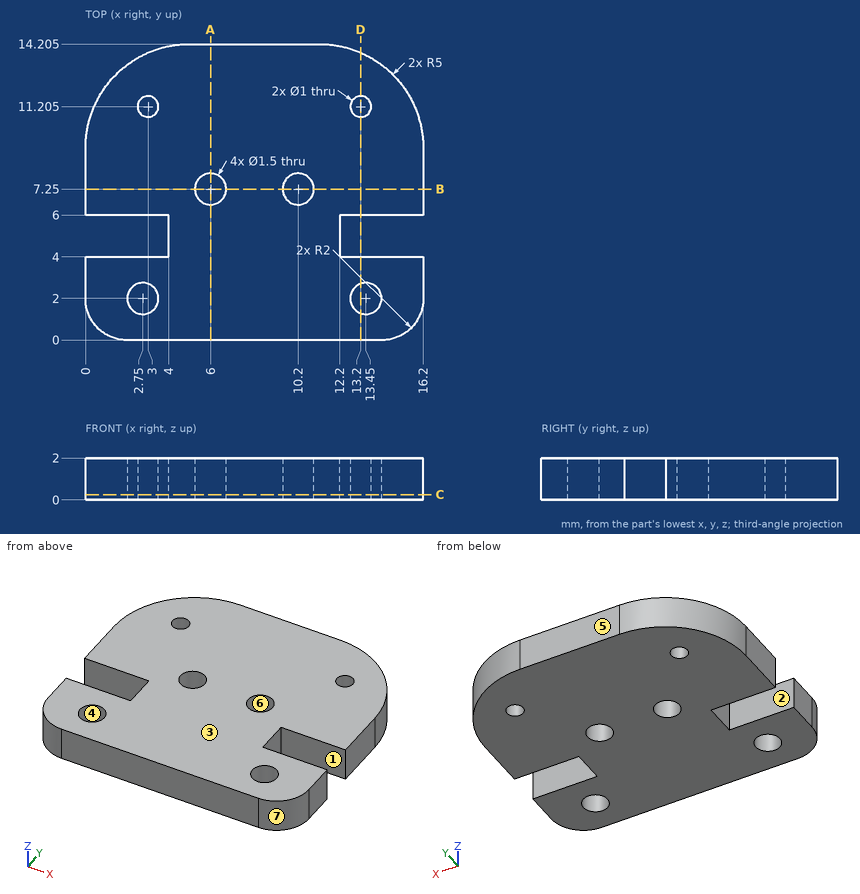
Here's the drawing with two shaded views (mm, measured from the low corner). I have some questions. A direction names the side the tool comes from. Coordinates: 2 decimals unless noted, no trailing zeros. Order: outer loops, then holes, each group sorted by start corner. A loop starts at its lowest first (then second) coordinate and runs counter-clockwise, first axis right, second up. Notation, with made-up numbers: M 5.5,64.25 L 21.5,64.25 A18 ccw 21.5,68.25 Z; hole C 60,61 d3. An arc over 180 degrees is marked long. Write item = value, one per line.
(1) For pin 1 Ø2 at (x, y) = (6, 7.25) entering from +Z; pin 2 Ø1 at (x, z) = (14, 0.5) entering from +Y; pin 3 Ø0.6 at (y, z) = (5, 1.5) entering from +X; pin 4 Ø1 at (x, z) = (3.5, 0.5) entering from +Y, each with a flat end and sliding along its axis, tell me the tip position at first contact or that it passes through.
Results are:
pin_1 = 2
pin_2 = 13.64
pin_3 = 12.2
pin_4 = 14.1
(2) I need wall thicknesses on line 1 along Y through (x, z) = (3, 0.6) (3 decimals); line 2 along Y through (x, z) = (6, 0.7) (3 decimals); line 3 along Y through (x, z) = (1.75, 1.8). Which ranges of each line are inside material? Lowest first, please. Write a range as [from, to].
Results are:
line_1 = [0, 1.293], [2.707, 4], [6, 10.705], [11.705, 13.788]
line_2 = [0, 6.5], [8, 14.205]
line_3 = [0.02, 4], [6, 13]
(3) Suppose I cut it at A-A on x = 6. Please give me the cut outline in (y, z) (3 decimals), plus the area to 3 significant figures.
Results are:
outline = M 0,0 L 6.5,0 L 6.5,2 L 0,2 Z; M 8,0 L 14.205,0 L 14.205,2 L 8,2 Z
area = 25.4 mm2
(4) Suppose I cut it at C-C on z = 0.25. Please give me the cut outline in (x, y) (3 decimals), plus the area to 3 significant figures.
Results are:
outline = M 0,2 A2 ccw 2,0 L 14.2,0 A2 ccw 16.2,2 L 16.2,4 L 12.2,4 L 12.2,6 L 16.2,6 L 16.2,9.205 A5 ccw 11.2,14.205 L 5,14.205 A5 ccw 0,9.205 L 0,6 L 4,6 L 4,4 L 0,4 Z; hole C 2.75,2 d1.5; hole C 3,11.205 d1; hole C 6,7.25 d1.5; hole C 10.2,7.25 d1.5; hole C 13.45,2 d1.5; hole C 13.2,11.205 d1
area = 193 mm2
(5) Suppose I cut it at D-D on x = 13.2. Please give me the cut outline in (y, z) (3 decimals), plus the area to 3 significant figures.
Results are:
outline = M 0,0 L 1.293,0 L 1.293,2 L 0,2 Z; M 2.707,0 L 4,0 L 4,2 L 2.707,2 Z; M 6,0 L 10.705,0 L 10.705,2 L 6,2 Z; M 11.705,0 L 13.788,0 L 13.788,2 L 11.705,2 Z
area = 18.7 mm2
(6) For the marked faces 1, 2 and 3, which set-ups out of +Z, -Z, +X, -X, +Y, -Y let a thin tool reach every point of the face, with its end or its side?
Results are:
face_1 = +Z, -Z, +X
face_2 = +Z, -Z, -X
face_3 = +Z, +X, -X, +Y, -Y
(7) If we mould it in two halves opening along Y, with no side actions, what happens to the marked faces 4, 5, 6 and 7? For each: pulls with the +Y half, pulls with the -Y half, needs draft (parallel to the pull), parting line crosses it, or undercut.
Results are:
face_4 = undercut
face_5 = pulls with the +Y half
face_6 = undercut
face_7 = pulls with the -Y half
(8) Suppose I cut it at B-B on y = 7.25. Please give me the cut outline in (x, z).
Results are:
outline = M 0,0 L 5.25,0 L 5.25,2 L 0,2 Z; M 6.75,0 L 9.45,0 L 9.45,2 L 6.75,2 Z; M 10.95,0 L 16.2,0 L 16.2,2 L 10.95,2 Z
